Verification items for the finished model (mm, model axes). Give positions to 0.01 mm unless a question says otherwise; leave off trailing zeros. Write each loop counter-clockwise with the first axis right and the second up, starting at its lowest first coordinate (ties: lowest second). Pieces come first, ordered by that corner, then holes.
from build123d import *

# Parameters (mm, degrees)
DISCO_START    = 3.175
CROQUIS1_R     = 15
DISCO_DEPTH    = 6.35
BARRENOS_START = 3.175
CROQUIS2_R     = 1.45
CROQUIS2_R_2   = 4
BARRENOS_DEPTH = 6.35


with BuildPart() as part:
    # Croquis1 → Disco (new body)
    with BuildSketch(Plane(origin=(0, 0, 0), x_dir=(1, 0, 0), z_dir=(0, 1, 0)).offset(DISCO_START)):
        with Locations(Location((152.4, -336.55, 0), (0, 0, 90))):
            Circle(CROQUIS1_R)
    extrude(amount=DISCO_DEPTH)

    # Croquis2 → Barrenos (cut)
    with BuildSketch(Plane(origin=(0, 0, 0), x_dir=(1, 0, 0), z_dir=(0, 1, 0)).offset(BARRENOS_START)):
        with Locations(Location((163.653984643, -341.990388742, 0), (0, 0, 90))):
            Circle(CROQUIS2_R)
        with Locations(Location((153.315477464, -349.016430965, 0), (0, 0, 90))):
            Circle(CROQUIS2_R)
        with Locations(Location((142.061492822, -343.576042223, 0), (0, 0, 90))):
            Circle(CROQUIS2_R)
        with Locations(Location((141.146015357, -331.109611258, 0), (0, 0, 90))):
            Circle(CROQUIS2_R)
        with Locations(Location((151.484522536, -324.083569035, 0), (0, 0, 90))):
            Circle(CROQUIS2_R)
        with Locations(Location((162.738507178, -329.523957777, 0), (0, 0, 90))):
            Circle(CROQUIS2_R)
        with Locations(Location((152.4, -336.55, 0), (0, 0, 90))):
            Circle(CROQUIS2_R_2)
    extrude(amount=BARRENOS_DEPTH, mode=Mode.SUBTRACT)


solid = part.part
Item 1: Release check for a two-part mould opening along Z. For faces 1 (the face through (156, 3.175, 333)), 2 (the face through (142.262, 6.306, 347.606)), 3 (the face through (152.34, 6.31, 350.09)) record: released by +Z, released by -Z, zero draft, split by the parting line, or undercut.
Answer key:
face 1: zero draft
face 2: split by the parting line
face 3: undercut
Item 2: Depth check by flat-ended pin: pin 1 (1.5 mm diameter, centred on x = 151, y = 6.5, fed in from +Z). Enter the tip coordinate at first touch or a pass-through.
Answer key:
pin 1: stops at z = 351.54
Item 3: Sectioned sample at A-A on z = 336.55. Record the cut outline in (x, y) (3 decimals).
Answer key:
outline: (137.4, 3.175) - (148.4, 3.175) - (148.4, 9.525) - (137.4, 9.525) - close; (156.4, 3.175) - (167.4, 3.175) - (167.4, 9.525) - (156.4, 9.525) - close
Item 4: Sectioned sample at B-B on x = 152.4. Record the cut outline in (y, z) (3 decimals), then the cut area to 3 significant figures.
Answer key:
outline: (3.175, 321.55) - (9.525, 321.55) - (9.525, 322.959) - (3.175, 322.959) - close; (3.175, 325.208) - (9.525, 325.208) - (9.525, 332.55) - (3.175, 332.55) - close; (3.175, 340.55) - (9.525, 340.55) - (9.525, 347.892) - (3.175, 347.892) - close; (3.175, 350.141) - (9.525, 350.141) - (9.525, 351.55) - (3.175, 351.55) - close
area: 111 mm2
Item 5: Sectioned sample at C-C on y = 7. Record the cut outline in (x, z).
Answer key:
outline: circle Ø30 at (152.4, 336.55); hole circle Ø2.9 at (141.15, 331.11); hole circle Ø2.9 at (142.06, 343.58); hole circle Ø8 at (152.4, 336.55); hole circle Ø2.9 at (151.48, 324.08); hole circle Ø2.9 at (153.32, 349.02); hole circle Ø2.9 at (162.74, 329.52); hole circle Ø2.9 at (163.65, 341.99)
Item 6: Sectioned sample at D-D on x = 155.5. Record the cut outline in (y, z) (3 decimals).
Answer key:
outline: (3.175, 321.874) - (9.525, 321.874) - (9.525, 334.022) - (3.175, 334.022) - close; (3.175, 339.078) - (9.525, 339.078) - (9.525, 351.226) - (3.175, 351.226) - close
Item 7: Scan lines: line 1 along Z through (x, y) = (162.5, 8); line 2 along Z through (x, y) = (152.4, 7); line 3 along X through (y, z) = (9, 336.5). Record each from-to range of solid material in increasing order.
Answer key:
line 1: z = 325.46 to 328.09, 330.95 to 341.11, 342.87 to 347.64
line 2: z = 321.55 to 322.96, 325.21 to 332.55, 340.55 to 347.89, 350.14 to 351.55
line 3: x = 137.4 to 148.4, 156.4 to 167.4
